The model under review builds one solid part; all positions refer to its coordinate system, in mm. Face numbers are marked on the shaded views. A direction names the side the tool comes from. Round coordinates to 2 decimals unless told otherwise and drop trailing zeros. Write each loop counter-clockwise with the first axis right and the second up, starting at its lowest first coordinate (ties: lowest second). Pieces come first, ordered by that corner, then holes. Notation, with made-up numbers: M 43.5,39 L 70.5,39 A18 cw 70.5,51 Z; hole C 33,44 d10. An arc over 180 degrees is marked long. One line per item, written item: value. Start each with the question number.
1) Take a section at C-C, the plane x = -3.25. Write out the cut boundary in (y, z) (3 decimals).
2) Take a section at D-D, the plane z = -1.5. Write out the cut boundary in (x, y).
3) Wall thickness on probe 1 along Z at (x, y) = (-1, 1.75); probe 2 along Y at (x, z) = (-1.75, -1); probe 3 along Y at (x, z) = (2, -1.75): over which ranges is each line inside the solid? List them lowest first.
4) Tool access review of the marked faces 1 and 2: name each direction out of +Z, -Z, +X, -X, +Y, -Y from which nothing blocks a thin tool from reaching the whole face with its end or side.
5) For P1, Ø0.5, axis at x = -4.5, z = 0.5, coming from the -Y side; P2, Ø3.5, axis at y = -1, z = -1.5, coming from the -X side; P3, Ø1.5, axis at y = -2, z = -0.5, coming from the +X side, all flat-tipped, find the tip position at first contact; note any pin that passes through.
6) Take a section at A-A, the plane x = -6.25. Write out the cut boundary in (y, z) (3 decimals), and give its area (3 significant figures).
Autodesk Inventor part; units mm, degrees
ref_plane "Work Plane1" through (0, 0, 0.25) normal (0, 0, -1) x (-1, 0, 0)
ref_plane "Work Plane2" through (0, 0, 0) normal (1, 0, 0) x (0, 0, -1)
ref_plane "YZ Plane" through (0, 0, 0) normal (1, 0, 0) x (0, 1, 0)
sketch "Sketch2" plane through (0, 0, 0) normal (0, 0, 1) x (1, 0, 0)
  line L0 (-9.3, 0) -> (9.3, 0)
  line L1 (9.3, 0) -> (9.3, 18.2)
  line L2 (9.3, 18.2) -> (-9.3, 18.2)
  line L3 (-9.3, 18.2) -> (-9.3, 0)
  point P0 (0, 0)
  point P1 (0, 0)
  dimension "d0" = 18.6
  dimension "d1" = 18.2
extrude "Extrusion1" add sketch "Sketch2" along normal blind 1
ref_plane "Work Plane1" through (0, 0, 0.25) normal (0, 0, -1) x (-1, 0, 0)
sketch "Sketch5" plane through (0, 0, 0) normal (0, 0, -1) x (-1, 0, 0)
  line L0 (-7.8, 6.7) -> (7.8, 6.7)
  line L1 (7.8, 6.7) -> (7.8, 16.7)
  line L2 (7.8, 16.7) -> (-7.8, 16.7)
  line L3 (-7.8, 16.7) -> (-7.8, 6.7)
  line L4 (9.3, 18.2) -> (9.3, 0)
  line L5 (9.3, 0) -> (-9.3, 0)
  line L6 (-9.3, 18.2) -> (9.3, 18.2)
  point P0 (0, 0)
  point P1 (0, 6.7)
  point P2 (0, 0)
  dimension "d13" = 10
  dimension "d15" = 1.5
  dimension "d16" = 1.5
ref_plane "Work Plane2" through (0, 0, 0) normal (1, 0, 0) x (0, 0, -1)
sketch "Sketch7" plane through (0, 0, 0) normal (1, 0, 0) x (0, 0, -1)
  arc A0 (-0.5, 0) -> (0.136, -1.4627) centre (1.5, 0) ccw
  line L0 (0, 0) -> (-1, 0)
  line L1 (0.136, -1.4627) -> (5.9868, -6.9187)
  line L2 (0, 18.2) -> (0, 0)
  line L3 (5.8504, -7.065) -> (-0.0004, -1.609)
  arc A1 (-0.7, 0) -> (-0.0004, -1.609) centre (1.5, 0) ccw
  line L4 (5.8504, -7.065) -> (5.9868, -6.9187)
  point P0 (5.9186, -6.9918)
  dimension "d19" = 2
  dimension "d22" = 43
  dimension "d23" = 0.5
  dimension "d24" = 0.2
  dimension "d33" = 8
extrude "Extrusion4" add sketch "Sketch7" along normal mid plane 10.3
sketch "Sketch8" plane through (0, 0, 0) normal (1, 0, 0) x (0, 0, -1)
  arc A0 (-0.5, 0) -> (0.136, -1.4627) centre (1.5, 0) ccw
  line L0 (-0.7, 0) -> (-0.5, 0)
  arc A1 (-0.7, 0) -> (-0.0004, -1.609) centre (1.5, 0) ccw construction
  line L1 (-0.0004, -1.609) -> (5.8504, -7.065)
  line L2 (5.8504, -7.065) -> (5.9868, -6.9187)
  line L3 (5.9868, -6.9187) -> (0.136, -1.4627)
  line L4 (2.1937, -3.655) -> (2.3301, -3.5087)
  point P0 (0, 0)
  dimension "d28" = 5
extrude "Extrusion5" add sketch "Sketch8" along normal mid plane 18.6
sketch "Sketch9" plane through (0, 0, 1) normal (0, 0, 1) x (1, 0, 0)
  line L0 (7.8, 16.7) -> (7.8, 6.7)
  line L1 (7.8, 6.7) -> (-7.8, 6.7)
  line L2 (-7.8, 6.7) -> (-7.8, 16.7)
  line L3 (-7.8, 16.7) -> (7.8, 16.7)
  point P0 (0, 0)
extrude "Extrusion6" add sketch "Sketch9" along normal blind 0.01
equation "\"BendRadius\" = Thickness"
equation "\"BendReliefWidth\" = Thickness"
equation "\"BendReliefDepth\" = 0.5 * Thickness"
equation "\"CornerReliefSize\" = 4 * Thickness"
equation "\"MinimumRemnant\" = 2 * Thickness"
equation "\"TransitionRadius\" = BendRadius"
equation "\"JacobiRadiusSize\" = BendRadius"
equation "\"GapSize\" = Thickness"
properties part number "0_42_oled"
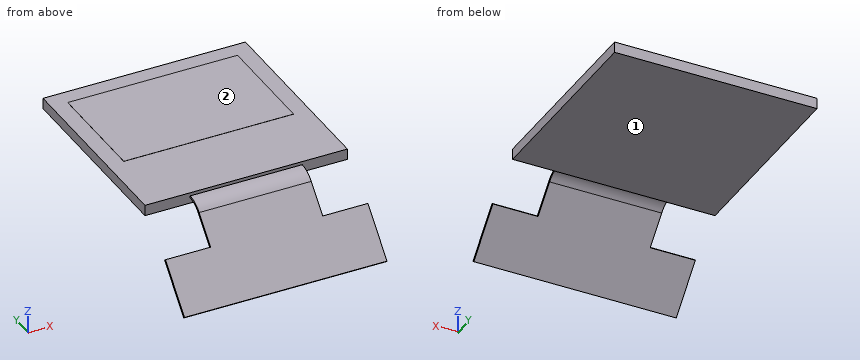
Checked values:
1. outline: M -7.065,-5.85 L -6.919,-5.987 L -1.463,-0.136 A2 cw 0,0.5 L 0,0 L 18.2,0 L 18.2,1 L 16.7,1 L 16.7,1.01 L 6.7,1.01 L 6.7,1 L 0,1 L 0,0.7 A2.2 ccw -1.609,0 Z
2. outline: M -5.15,-3.01 L 5.15,-3.01 L 5.15,-2.73 L -5.15,-2.73 Z
3. probe 1: z = 0 to 1
3. probe 2: y = -2.54 to -2.27
3. probe 3: y = -3.24 to -2.97
4. face 1: -Z, +X, -X, +Y
4. face 2: +Z, +X, -X, +Y, -Y
5. P1: stops at y = -1.33
5. P2: stops at x = -5.15
5. P3: stops at x = 5.15
6. outline: M -7.065,-5.85 L -6.919,-5.987 L -3.509,-2.33 L -3.655,-2.194 Z; M 0,0 L 18.2,0 L 18.2,1 L 16.7,1 L 16.7,1.01 L 6.7,1.01 L 6.7,1 L 0,1 Z
6. area: 19.3 mm2
